Build history of the part. All positions in model axes, mm. Face numbers are marked on the shaded views. A direction names the side the tool comes from. Give positions to 0.01 mm unless a question says otherwise; leave off trailing zeros. Loops run counter-clockwise (first coordinate to the right, second up) from the corner with the lowest first, then second, coordinate; pieces in that order, holes last. Notation, with made-up numbers: (-26, 75) - (27, 75) arc R6 ccw to (27, 86) - close; hole circle Ø11 at (-38.5, 44). An arc over 180 degrees is marked (long way). Return JSON: item names as keys, results as strings. Group by question number.
1) Slice it at C-C (x = 65.5). List the corners of the cut face in (y, z), and give its area (3 significant figures).
2) Slice it at B-B (x = 41). List the corners of the cut face in (y, z).
3) Mould opens along X. For the marked faces 3, 4, 5 and 6 say: released by +X, released by -X, zero draft, split by the parting line, or undercut.
4) 3-axis set-ups, long thin cutter, end or side, ignore diameter. For the marked faces 1 and 2: which of +Z, -Z, +X, -X, +Y, -Y reach the whole face in a straight line?
5) Slice it at A-A (z = 41). List the corners of the cut face in (x, y).
6) Drop flat-ended pins along their axis: pin 1 (10 mm diameter, centred on x = -10.5, y = -14.5, fed in from +Z); pin 2 (4 mm diameter, centred on x = -35, y = 6, fed in from +Z); pin 3 (1.5 mm diameter, centred on x = 23.5, y = -37.5, fed in from -Z). Give the stop position or say it passes through.
7) Drill centre lines: probe 1 along X at (y, z) = (-5.5, 35); probe 2 along Y at (x, z) = (42.5, 28); probe 3 along Z at (x, y) = (30, 45.5). Where is each one in solid material? Low to high. Write a range as from..to.
8) Slice it at D-D (y = 19). List the corners of the cut face in (x, z).
```python
from build123d import *

# Parameters (mm, degrees)
SKETCH_1_W          = 111
SKETCH_1_H          = 91
SKETCH_1_W_2        = 101
SKETCH_1_H_2        = 81
EXTRUDE_1_DEPTH     = 46
SKETCH_2_W          = 111
SKETCH_2_H          = 91
EXTRUDE_2_DEPTH     = 5
SKETCH_3_W          = 101
SKETCH_3_H          = 26
CUT_EXTRUDE_1_DEPTH = 5
FILLET_1_R          = 2
SKETCH_4_W          = 5
SKETCH_4_H          = 10
CUT_EXTRUDE_2_DEPTH = 15
SKETCH_5_W          = 81
SKETCH_5_H          = 5
CUT_EXTRUDE_3_DEPTH = 5


with BuildPart() as part:
    # 草圖1 → 填料-伸長1 (new body)
    with BuildSketch(Plane.XY):
        with Locations((18.39111128, 6.255540432)):
            Rectangle(SKETCH_1_W, SKETCH_1_H)
        with Locations((18.39111128, 6.255540432)):
            Rectangle(SKETCH_1_W_2, SKETCH_1_H_2, mode=Mode.SUBTRACT)
    extrude(amount=EXTRUDE_1_DEPTH)

    # 草圖2 → 填料-伸長2 (add)
    with BuildSketch(Plane(origin=(0, 0, 0), x_dir=(-1, 0, 0), z_dir=(0, 0, -1))):
        with Locations((-18.39111128, 6.255540432)):
            Rectangle(SKETCH_2_W, SKETCH_2_H)
    extrude(amount=EXTRUDE_2_DEPTH)

    # 草圖3 → 除料-伸長1 (cut)
    with BuildSketch(Plane.XZ.offset(39.244459568)):
        with Locations((18.39111128, 8)):
            Rectangle(SKETCH_3_W, SKETCH_3_H)
    extrude(amount=-CUT_EXTRUDE_1_DEPTH, mode=Mode.SUBTRACT)

    # 圓角1
    fillet_1_edges = [part.edges().sort_by_distance(p)[0] for p in [
        (18.39111128, -34.244459568, 0),
    ]]
    fillet(fillet_1_edges, radius=FILLET_1_R)

    # 草圖4 → 除料-伸長2 (cut)
    with BuildSketch(Plane.XY.offset(46)):
        with Locations((-34.60888872, 6.755540432)):
            Rectangle(SKETCH_4_W, SKETCH_4_H)
        with Locations((71.39111128, 6.755540432)):
            Rectangle(SKETCH_4_W, SKETCH_4_H)
    extrude(amount=-CUT_EXTRUDE_2_DEPTH, mode=Mode.SUBTRACT)

    # 草圖5 → 除料-伸長3 (cut)
    with BuildSketch(Plane(origin=(0, 51.755540432, 0), x_dir=(1, 0, 0), z_dir=(0, 1, 0))):
        with Locations((18.39111128, -22.5)):
            Rectangle(SKETCH_5_W, SKETCH_5_H)
        with Locations((18.39111128, -12.5)):
            Rectangle(SKETCH_5_W, SKETCH_5_H)
    extrude(amount=-CUT_EXTRUDE_3_DEPTH, mode=Mode.SUBTRACT)


solid = part.part
```
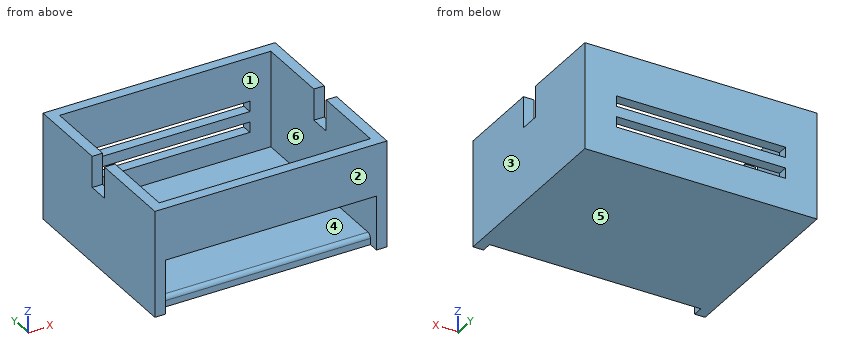
Results:
{
 "1": {"outline": "(-39.24, 21) - (-34.24, 21) - (-34.24, 46) - (-39.24, 46) - close; (-34.24, -5) - (51.76, -5) - (51.76, 46) - (46.76, 46) - (46.76, 0) - (-32.24, 0) arc R2 ccw to (-34.24, -2) - close", "area": "784 mm2"},
 "2": {"outline": "(-39.24, 21) - (-34.24, 21) - (-34.24, 46) - (-39.24, 46) - close; (-34.24, -5) - (51.76, -5) - (51.76, 10) - (46.76, 10) - (46.76, 0) - (-32.24, 0) arc R2 ccw to (-34.24, -2) - close; (46.76, 15) - (51.76, 15) - (51.76, 20) - (46.76, 20) - close; (46.76, 25) - (51.76, 25) - (51.76, 46) - (46.76, 46) - close"},
 "3": {"face 3": "released by +X", "face 4": "undercut", "face 5": "zero draft", "face 6": "undercut"},
 "4": {"face 1": "+Z", "face 2": "+Z, -Z, +X, -X, -Y"},
 "5": {"outline": "(-37.11, -39.24) - (73.89, -39.24) - (73.89, 1.76) - (68.89, 1.76) - (68.89, -34.24) - (-32.11, -34.24) - (-32.11, 1.76) - (-37.11, 1.76) - close; (-37.11, 11.76) - (-32.11, 11.76) - (-32.11, 46.76) - (68.89, 46.76) - (68.89, 11.76) - (73.89, 11.76) - (73.89, 51.76) - (-37.11, 51.76) - close"},
 "6": {"pin 1": "z = 0", "pin 2": "z = 31", "pin 3": "z = 21"},
 "7": {"probe 1": "-37.11..-32.11, 68.89..73.89", "probe 2": "-39.24..-34.24, 46.76..51.76", "probe 3": "-5..0"},
 "8": {"outline": "(-37.11, -5) - (73.89, -5) - (73.89, 46) - (68.89, 46) - (68.89, 0) - (-32.11, 0) - (-32.11, 46) - (-37.11, 46) - close"}
}
